Can you work these out from the model? Positions are in its coordinate system, mm. Give positions to 0.01 mm unless a question says otherwise; leave off trailing zeros. Order: outer loops, then holes, each group sorted by start corner. A loop starts at its lowest first (then second) coordinate and runs counter-clockwise, first axis right, second up. Notation, with made-up numbers: (79.5, 27.5) -> (83.5, 27.5) arc R17 ccw to (83.5, 52.5) -> close; hole circle Ø5 at (28.5, 68.5). An arc over 180 degrees is marked (long way). Answer as CSV lines item,"result".
```python
from build123d import *

# Parameters (mm, degrees)
F1_DEPTH = 4.7625


with BuildPart() as f1:
    # F0 (on Top) → F1 (new body)
    with BuildSketch(Plane.XY):
        with BuildLine():
            ThreePointArc((0, 9.117891), (-5.189841, 9.689006), (-10.209356, 8.251961))
            Line((-10.209356, 8.251961), (-12.369341, 7.146457))
            Line((-12.369341, 7.146457), (-12.369341, 4.638605))
            ThreePointArc((-12.369341, 4.638605), (-11.185748, -0.503205), (-7.873208, -4.610051))
            ThreePointArc((-7.873208, -4.610051), (-5.859185, -9.348483), (-2.140938, -12.909897))
            Line((-2.140938, -12.909897), (0, -14.256157))
            Line((0, -14.256157), (1.969674, -12.909897))
            ThreePointArc((1.969674, -12.909897), (5.637264, -9.298956), (7.81588, -4.635937))
            ThreePointArc((7.81588, -4.635937), (10.7633, -0.362437), (12.15602, 4.638605))
            Line((12.15602, 4.638605), (12.15602, 7.146457))
            Line((12.15602, 7.146457), (9.996034, 8.251961))
            ThreePointArc((9.996034, 8.251961), (5.082776, 9.663363), (0, 9.117891))
        make_face()
    extrude(amount=F1_DEPTH)


solid = f1.part
```
Item 1: Imagine slicing it at B-B, the plane x = 6. Please give me the cut outline in (y, z), then the cut area to 3 significant figures.
Numbers:
outline,"(-8.76, 0) -> (9.55, 0) -> (9.55, 4.76) -> (-8.76, 4.76) -> close"
area,"87.2 mm²"
Item 2: Please list where these lines run through material, in increasing order: line 1 along X through (y, z) = (-2.75, 1.75); line 2 along X through (y, z) = (0.75, 2.9); line 3 along Y through (x, z) = (-6, 1.65).
Numbers:
line 1,"x = -9.76 to 9.38"
line 2,"x = -11.71 to 11.23"
line 3,"y = -9.14 to 9.6"
Item 3: Imagine slicing it at C-C, the plane y = -6.5. Please give me the cut outline in (x, z).
Numbers:
outline,"(-7.34, 0) -> (7.18, 0) -> (7.18, 4.76) -> (-7.34, 4.76) -> close"
Item 4: For pin 1 (1.5 mm diameter, centred on y = -10.5, z = 3, fed in from +X); pin 2 (1.5 mm diameter, centred on x = 2, z = 3.5, fed in from -Y), each with a flat end and sliding along its axis, tell me the tip position at first contact or that it passes through.
Numbers:
pin 1,"stops at x = 5.31"
pin 2,"stops at y = -13.4"
Item 5: We'd pull the mould along X, two halves only. Please class faces 1 (the cylindrical face through (5.595, -9.358, 2.348)), 2 (the cylindrical face through (-11.218, -0.436, 2.348)), 3 (the cylindrical face through (5.155, 9.657, 2.348)): released by +X, released by -X, zero draft, split by the parting line, or undercut.
Numbers:
face 1,"released by +X"
face 2,"released by -X"
face 3,"undercut"
Item 6: Imagine slicing it at A-A, the plane z = 2.65. Please give me the cut outline in (x, y).
Numbers:
outline,"(-12.37, 4.64) arc R11.76 ccw to (-7.87, -4.61) arc R12.8 ccw to (-2.14, -12.91) -> (0, -14.26) -> (1.97, -12.91) arc R14.53 ccw to (7.82, -4.64) arc R15.7 ccw to (12.16, 4.64) -> (12.16, 7.15) -> (10, 8.25) arc R13.3 ccw to (0, 9.12) arc R13.53 ccw to (-10.21, 8.25) -> (-12.37, 7.15) -> close"
